Geometry check sheet. Reference: the model listing, model coordinates, mm. Give positions to 0.01 mm unless a question says otherwise; leave off trailing zeros. Loops run counter-clockwise (first coordinate to the right, second up) from the corner with the lowest first, then second, coordinate; pieces in that order, holes last.
1. Cross-section at A-A, the plane x = 28.5. Record the cut outline in (y, z).
2. Cross-section at C-C, the plane z = 17.25. Record the cut outline in (x, y), plus the area to 3 significant figures.
3. Release check for a two-part mould opening along Y. For faces 1 (the cylindrical face through (0.451, -19.757, 9.86)), 2 (the cylindrical face through (-32.3, -43.58, 9.86)), 3 (the flat face through (-2, 19, 0)) record: +Y half, -Y half, draft (parallel to the pull), parting line (faces both ways), or undercut.
4. Cross-section at D-D, the plane y = 35. Record the cut outline in (x, z), plus the area to 3 significant figures.
5. Cross-section at B-B, the plane y = -8. Record the cut outline in (x, z).
6. Go/stop test with flat-tipped pins: pin 1 Ø2 at (y, z) = (24, 5.5) entering from +X; pin 2 Ø6 at (y, z) = (-29, 18) entering from +X; pin 3 Ø12 at (y, z) = (-10.5, 6) entering from +X. Record where each tip stops, or that it passes through.
7. Material ranges on L1, parallel to X at y = -6, z = 7.5; L2, parallel to X at y = -17, z = 16; L3, parallel to Y at x = -32, z = 1.5, recorded low to high.
from build123d import *

# Parameters (mm, degrees)
SKETCH_R  = 18.849926
PAD_DEPTH = 20


with BuildPart() as part:
    # Sketch → Pad (new body)
    with BuildSketch(Plane.XY):
        with BuildLine():
            ThreePointArc((6.009813, 43.763913), (-2.307048, 53.935241), (-8.940587, 42.594066))
            ThreePointArc((-38.571066, 19.895965), (-14.659471, 19.370481), (-8.940587, 42.594066))
            ThreePointArc((-38.571066, 19.895965), (-51.372493, 16.065234), (-42.79749, 5.81729))
            ThreePointArc((-31.512922, -29.994656), (-22.378417, -7.432425), (-42.79749, 5.81729))
            ThreePointArc((-31.512922, -29.994656), (-32.109292, -43.708122), (-19.737971, -37.761257))
            ThreePointArc((19.745172, -37.841497), (0.040281, -19.752175), (-19.737971, -37.761257))
            ThreePointArc((19.745172, -37.841497), (32.535801, -43.526638), (30.567408, -29.668556))
            ThreePointArc((39.530273, 8.579484), (18.337441, -6.628465), (30.567408, -29.668556))
            ThreePointArc((39.530273, 8.579484), (48.01508, 18.640488), (35.605471, 23.024247))
            ThreePointArc((6.009813, 43.763913), (13.423393, 22.856702), (35.605471, 23.024247))
        make_face()
        Circle(SKETCH_R, mode=Mode.SUBTRACT)
    extrude(amount=PAD_DEPTH)


solid = part.part
Result:
1. outline: (-45.1, 0) - (-28.74, 0) - (-28.74, 20) - (-45.1, 20) - close; (6.44, 0) - (19.84, 0) - (19.84, 20) - (6.44, 20) - close
2. outline: (-42.8, 5.82) arc R19.12 cw to (-31.51, -29.99) arc R8 ccw (long way) to (-19.74, -37.76) arc R19.82 cw to (19.75, -37.84) arc R8 ccw (long way) to (30.57, -29.67) arc R19.82 cw to (39.53, 8.58) arc R8 ccw (long way) to (35.61, 23.02) arc R19.12 cw to (6.01, 43.76) arc R8 ccw (long way) to (-8.94, 42.59) arc R19.12 cw to (-38.57, 19.9) arc R8 ccw (long way) to start; hole circle Ø37.7 at (0, 0)
2. area: 2,560 mm2
3. face 1: -Y half
3. face 2: undercut
3. face 3: draft
4. outline: (-7.17, 0) - (5.6, 0) - (5.6, 20) - (-7.17, 20) - close
4. area: 255 mm2
5. outline: (-22.21, 0) - (-17.07, 0) - (-17.07, 20) - (-22.21, 20) - close; (17.07, 0) - (18.07, 0) - (18.07, 20) - (17.07, 20) - close
6. pin 1: stops at x = 45.02
6. pin 2: stops at x = 33.84
6. pin 3: stops at x = 18.96
7. L1: x = -22.89 to -17.87, 17.87 to 18.5
7. L2: x = -21.88 to -8.14, 8.14 to 18.7
7. L3: y = -43.78 to -30.28, 3.89 to 16.3
